from build123d import *

# Parameters (mm, degrees)
F0_W     = 1.5748
F0_H     = 38.1
F1_DEPTH = 4.7498
F2_SIZE  = 0.762


# Not quite as in the source:
# - a feature names something its author has since deleted; it is built from what else it names


with BuildPart() as f1:
    # F0 (on Top) → F1 (new body)
    with BuildSketch(Plane.XY):
        with Locations((-11.2433909576, -6.3634803519)):
            Rectangle(F0_W, F0_H)
        with BuildLine():
            Line((-10.4559909576, -25.4134803519), (-12.0307909576, -25.4134803519))
            Line((-12.0307909576, -25.4134803519), (-12.0307909576, 12.6865196481))
            Line((-12.0307909576, 12.6865196481), (-12.0307909576, 17.1203389764))
            Line((-12.0307909576, 17.1203389764), (-13.6055909576, 12.6865196481))
            Line((-13.6055909576, 12.6865196481), (-13.6055909576, -25.4134803519))
            Line((-13.6055909576, -25.4134803519), (-18.3553909576, -25.4134803519))
            Line((-18.3553909576, -25.4134803519), (-18.3553909576, -27.7027830635))
            ThreePointArc((-18.3553909576, -27.7027830635), (-17.6114421818, -29.4988342878), (-15.8153909576, -30.2427830635))
            Line((-15.8153909576, -30.2427830635), (20.3288090424, -30.2427830635))
            ThreePointArc((20.3288090424, -30.2427830635), (22.1248602666, -29.4988342878), (22.8688090424, -27.7027830635))
            Line((22.8688090424, -27.7027830635), (22.8688090424, -25.4134803519))
            Line((22.8688090424, -25.4134803519), (18.1190090424, -25.4134803519))
            Line((18.1190090424, -25.4134803519), (18.1190090424, 12.6865196481))
            Line((18.1190090424, 12.6865196481), (16.5442090424, 17.1203389764))
            Line((16.5442090424, 17.1203389764), (16.5442090424, 12.6865196481))
            Line((16.5442090424, 12.6865196481), (16.5442090424, -25.4134803519))
            Line((16.5442090424, -25.4134803519), (14.9694090424, -25.4134803519))
            Line((14.9694090424, -25.4134803519), (-10.4559909576, -25.4134803519))
        make_face()
        with Locations((15.7568090424, -6.3634803519)):
            Rectangle(F0_W, F0_H)
        Polygon((-12.0307909576, 17.1203389764), (-12.0307909576, 12.6865196481), (-10.4559909576, 12.6865196481), align=None)
        Polygon((16.5442090424, 17.1203389764), (14.9694090424, 12.6865196481), (16.5442090424, 12.6865196481), align=None)
    extrude(amount=F1_DEPTH)

    # F2
    f2_edges = [f1.edges().sort_by_distance(p)[0] for p in [
        (-13.605591, -6.36348, 4.7498),
        (-10.455991, -6.36348, 4.7498),
        (-11.243391, 14.903429, 4.7498),
        (-12.818191, 14.903429, 4.7498),
        (-15.980491, -25.41348, 4.7498),
        (-18.355391, -26.558132, 4.7498),
        (-17.611442, -29.498834, 4.7498),
        (2.256709, -30.242783, 4.7498),
        (22.12486, -29.498834, 4.7498),
        (22.868809, -26.558132, 4.7498),
        (20.493909, -25.41348, 4.7498),
        (18.119009, -6.36348, 4.7498),
        (17.331609, 14.903429, 4.7498),
        (15.756809, 14.903429, 4.7498),
        (14.969409, -6.36348, 4.7498),
        (2.256709, -25.41348, 4.7498),
        (-10.455991, -6.36348, 0),
        (-11.243391, 14.903429, 0),
        (-12.818191, 14.903429, 0),
        (-13.605591, -6.36348, 0),
        (-15.980491, -25.41348, 0),
        (-18.355391, -26.558132, 0),
        (-17.611442, -29.498834, 0),
        (2.256709, -30.242783, 0),
        (22.12486, -29.498834, 0),
        (22.868809, -26.558132, 0),
        (20.493909, -25.41348, 0),
        (18.119009, -6.36348, 0),
        (17.331609, 14.903429, 0),
        (15.756809, 14.903429, 0),
        (14.969409, -6.36348, 0),
        (2.256709, -25.41348, 0),
    ]]
    chamfer(f2_edges, length=F2_SIZE)


solid = f1.part
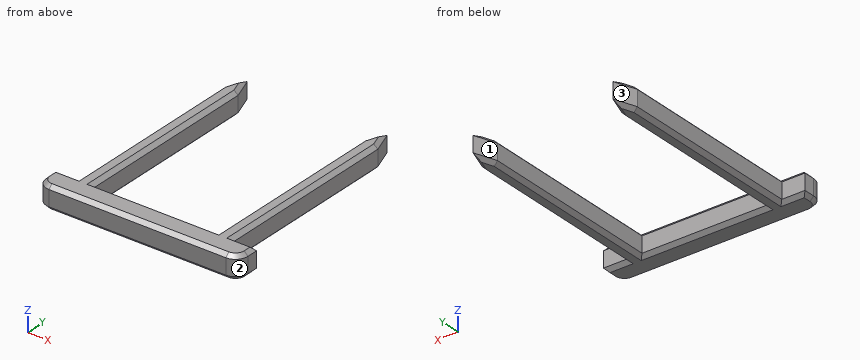
Could you check a few things on this model? Use its own coordinates, in mm. Face numbers are marked on the shaded views. Give positions to 0.01 mm unless a question says otherwise; leave off trailing zeros. Order: outer loops, then holes, each group sorted by start corner. A loop starts at its lowest first (then second) coordinate and runs counter-clockwise, first axis right, second up. Notation, with made-up numbers: (7, 59.25) -> (32, 59.25) arc R19 cw to (32, 66.25) -> close; hole circle Ø4 at (-14.75, 45.25). An arc over 180 degrees is marked (long way). Answer in a Markdown table with one row per item. Add a question column.
Item 1: Imagine slicing it at C-C (z = 2.5). List the corners of the cut face in (x, y) for me, and give its area (3 significant figures).
Item 2: We'd pull the mould along X, two halves only. Please class the marked faces 1, 2 and 3: pulls with the +X half, pulls with the -X half, needs draft (parallel to the pull), parting line crosses it, or undercut.
Item 3: Imagine slicing it at B-B (y = 8). List the corners of the cut face in (x, z) for me, and give its area (3 significant figures).
Item 4: I'm going to push flat-ended pins straight in: P1, Ø1, axis at x = 4.5, z = 2, coming from the +Y side; P2, Ø1.6, axis at y = -13, z = 2, coming from the +X side; P3, Ø2.5, axis at y = -2.5, z = 1.5, coming from the -X side. Where does each tip first touch, or does it pass through?
Item 5: Please list where these lines run through material, in increasing order: probe 1 along X at (y, z) = (-1.5, 1.85); probe 2 along Y at (x, z) = (7.5, 3.7); probe 3 along X at (y, z) = (14, 2.8).
Item 6: Imagine slicing it at A-A (x = 7). List the corners of the cut face in (y, z) for me, and give its area (3 significant figures).
Result:
| question | item | result |
|---|---|---|
| 1 | outline | (-18.36, -27.7) arc R2.54 ccw to (-15.82, -30.24) -> (20.33, -30.24) arc R2.54 ccw to (22.87, -27.7) -> (22.87, -25.41) -> (18.12, -25.41) -> (18.12, 12.69) -> (16.54, 17.12) -> (14.97, 12.69) -> (14.97, -25.41) -> (-10.46, -25.41) -> (-10.46, 12.69) -> (-12.03, 17.12) -> (-13.61, 12.69) -> (-13.61, -25.41) -> (-18.36, -25.41) -> close |
| 1 | area | 450 mm2 |
| 2 | face 1 | undercut |
| 2 | face 2 | pulls with the +X half |
| 2 | face 3 | pulls with the -X half |
| 3 | outline | (-13.61, 0.76) -> (-12.84, 0) -> (-11.22, 0) -> (-10.46, 0.76) -> (-10.46, 3.99) -> (-11.22, 4.75) -> (-12.84, 4.75) -> (-13.61, 3.99) -> close; (14.97, 0.76) -> (15.73, 0) -> (17.36, 0) -> (18.12, 0.76) -> (18.12, 3.99) -> (17.36, 4.75) -> (15.73, 4.75) -> (14.97, 3.99) -> close |
| 3 | area | 27.6 mm2 |
| 4 | P1 | y = -25.41 |
| 4 | P2 | x = 18.12 |
| 4 | P3 | x = -13.61 |
| 5 | probe 1 | -13.61 to -10.46, 14.97 to 18.12 |
| 5 | probe 2 | -30.24 to -25.41 |
| 5 | probe 3 | -13.14 to -10.92, 15.44 to 17.65 |
| 6 | outline | (-30.24, 0.76) -> (-29.48, 0) -> (-26.18, 0) -> (-25.41, 0.76) -> (-25.41, 3.99) -> (-26.18, 4.75) -> (-29.48, 4.75) -> (-30.24, 3.99) -> close |
| 6 | area | 21.8 mm2 |
